from build123d import *

# Parameters (mm, degrees)
F1_DEPTH = 10
F2_R     = 2
F3_DEPTH = 25
F4_R     = 3


with BuildPart() as f1:
    # F0 (on Top) → F1 (new body)
    with BuildSketch(Plane.XY):
        Polygon((0, 2), (0, 0), (15, 0), (15, 10), (22.25, 10), (29.5, 10), (29.5, 0), (44.5, 0), (44.5, 2), (31.5, 2), (31.5, 12), (22.25, 12), (13, 12), (13, 2), align=None)
    extrude(amount=F1_DEPTH)

    # F2 (on face) → F3 (cut)
    with BuildSketch(Plane(origin=(0, 2, 0), x_dir=(-1, 0, 0), z_dir=(0, 1, 0))):
        with Locations((-38, 5)):
            Circle(F2_R)
        with Locations((-6.5, 5)):
            Circle(F2_R)
    extrude(amount=-F3_DEPTH, mode=Mode.SUBTRACT)

    # F4
    f4_edges = [f1.edges().sort_by_distance(p)[0] for p in [
        (31.5, 2, 5),
        (13, 2, 5),
        (29.5, 0, 5),
        (15, 0, 5),
    ]]
    fillet(f4_edges, radius=F4_R)


solid = f1.part
CAD build for the part. Positions are in the model's coordinates, mm. A direction names the side the tool comes from. Round coordinates to 2 decimals unless told otherwise and drop trailing zeros. Write each loop counter-clockwise with the first axis right and the second up, starting at its lowest first coordinate (ties: lowest second). Pieces come first, ordered by that corner, then holes. Notation, with made-up numbers: M 27.5,29.25 L 77.5,29.25 A24 cw 77.5,65.25 Z; hole C -17.75,16.25 d1. An arc over 180 degrees is marked long. Put each result on its own line as item: value. Start each with the question number.
1) Saw through at D-D, the plane z = 8.75. Write the cut outline in (x, y), and give its area (3 significant figures).
2) Saw through at C-C, the plane y = 1. Write the cut outline in (x, z), and give its area (3 significant figures).
3) Pin check, flat tips, straight feed: pin 1 Ø3 at (x, z) = (41, 6.5) entering from +Y; pin 2 Ø3.5 at (y, z) = (5.5, 5.5) entering from +X; pin 3 Ø5.5 at (y, z) = (7.5, 3) entering from -X. Stop position of each tip, or through.
4) 3-axis set-ups, long thin cutter, end or side, ignore diameter. For faces 4 (the flat face through (41, 2, 5)), 5 (the flat face through (4, 2, 5)), 6 (the flat face through (15, 6, 5)), 7 (the flat face through (22, 12, 5)): which of +Z, -Z, +X, -X, +Y, -Y reach the whole face in a straight line?
5) Saw through at B-B, the plane x = 6.5. Write the cut outline in (y, z), and give its area (3 significant figures).
6) Pull direction Z, two halves, no side cores. Call faces 1 (the flat face through (20.5, 10.5, 10)), 2 (the cylindrical face through (8.498, 1.014, 5.088)), 3 (the flat face through (0, 1, 5)): pulls with the +Z half, pulls with the -Z half, needs draft (parallel to the pull), parting line crosses it, or undercut.
7) Saw through at A-A, the plane y = 6.75. Write the cut outline in (x, z), and give its area (3 significant figures).
8) Drill centre lines: probe 1 along X at (y, z) = (5.75, 5.5); probe 2 along Z at (x, y) = (6.5, 1.25); probe 3 along X at (y, z) = (1.25, 3.25). Where is each one in solid material? Low to high. Write a range as [from, to].
Resolved:
1. outline: M 0,0 L 12,0 A3 ccw 15,3 L 15,10 L 29.5,10 L 29.5,3 A3 ccw 32.5,0 L 44.5,0 L 44.5,2 L 34.5,2 A3 cw 31.5,5 L 31.5,12 L 13,12 L 13,5 A3 cw 10,2 L 0,2 Z
1. area: 129 mm²
2. outline: M 0,0 L 14.24,0 L 14.24,10 L 0,10 Z; M 30.26,0 L 44.5,0 L 44.5,10 L 30.26,10 Z; hole C 6.5,5 d4; hole C 38,5 d4
2. area: 260 mm²
3. pin 1: y = 2
3. pin 2: x = 31.77
3. pin 3: x = 12.99
4. face 4: +Z, -Z, +X, +Y
4. face 5: +Z, -Z, -X, +Y
4. face 6: +Z, -Z, -Y
4. face 7: +Z, -Z, +X, -X, +Y
5. outline: M 0,0 L 2,0 L 2,3 L 0,3 Z; M 0,7 L 2,7 L 2,10 L 0,10 Z
5. area: 12.0 mm²
6. face 1: pulls with the +Z half
6. face 2: undercut
6. face 3: needs draft
7. outline: M 13,0 L 15,0 L 15,10 L 13,10 Z; M 29.5,0 L 31.5,0 L 31.5,10 L 29.5,10 Z
7. area: 40.0 mm²
8. probe 1: [13, 15], [29.5, 31.5]
8. probe 2: [0, 3], [7, 10]
8. probe 3: [0, 5.53], [7.47, 14.44], [30.06, 37.03], [38.97, 44.5]
